Geometry check sheet. Reference: the model listing, model coordinates, mm. Face numbers are marked on the shaded views. A direction names the side the tool comes from. Coordinates: 2 decimals unless noted, no trailing zeros. Write each loop counter-clockwise with the first axis right and the second up, starting at its lowest first coordinate (ties: lowest second). Pieces come first, ordered by that corner, then holes. Notation, with made-up numbers: (49.25, 85) -> (58.25, 85) arc R13 ccw to (58.25, 90) -> close; hole circle Ø11 at (-34, 45.5). An arc over 180 degrees is marked (long way). Answer in a Markdown table with one row per item. Add a question column.
1. Set-up check for the marked faces 1, 2, 3, 4 and 5: record each of +Z, -Z, +X, -X, +Y, -Y from which the full face is reachable in a straight line by a thin tool's end or side.
2. Depth check by flat-ended pin: P1, Ø2, axis at x = 19, z = -17, coming from the -Y side; P2, Ø5.5, axis at x = 6.5, z = -15, coming from the +Y side; P3, Ø1.8, axis at x = -30, z = -1, coming from the +Y side; P4, Ø4, axis at y = -35.36, z = -35.36, coming from the +X side. Enter the tip coordinate at first touch or a pass-through.
3. Cross-section at D-D on y = 22. Record the cut outline in (x, z).
4. Cross-section at B-B on x = 175.7. Record the cut outline in (y, z), and give its area (3 significant figures).
5. Scan lines: L1, parallel to X at y = 43, z = 0; L2, parallel to X at y = 50.5, z = 0; L3, parallel to Z at x = 128.5, y = 24. Record each from-to range of solid material in increasing order. Write a range as from..to.
6. Cross-section at C-C on y = -27. Record the cut outline in (x, z), and give its area (3 significant figures).
7. Cross-section at A-A on z = -19. Record the cut outline in (x, y), and give its area (3 significant figures).
8. Mould release check, pull along X, two halves, no side actions. Record for the marked faces 6, 7 and 8: pulls with the +X half, pulls with the -X half, needs draft (parallel to the pull), parting line crosses it, or undercut.
```python
from build123d import *

# Parameters (mm, degrees)
BOSS_EXTRUDE1_DEPTH      = 10
BOSS_EXTRUDE1_DEPTH_BACK = 38
SKETCH1_3_R              = 40
BOSS_EXTRUDE2_DEPTH      = 10
SKETCH1_4_R              = 45
SKETCH1_4_R_2            = 40
BOSS_EXTRUDE3_DEPTH      = 9
SKETCH2_R                = 45
SKETCH2_W                = 60
SKETCH2_H                = 60
BOSS_EXTRUDE4_DEPTH      = 30
SKETCH2_3_W              = 60
SKETCH2_3_H              = 60
BOSS_EXTRUDE5_DEPTH      = 205.7
SKETCH3_W                = 60
SKETCH3_H                = 60
SKETCH3_R                = 7
BOSS_EXTRUDE6_DEPTH      = 60.5
CHAMFER1_SIZE            = 25
BOSS_EXTRUDE7_DEPTH      = 11
SKETCH7_R                = 3.25
CUT_EXTRUDE2_DEPTH       = 51


with BuildPart() as part:
    # Sketch1 → Boss-Extrude1 (new, two sides: drawn at the far end of the back side and taken through both)
    with BuildSketch(Plane(origin=(0, 0, 0), x_dir=(0, 0, -1), z_dir=(1, 0, 0)).offset(-BOSS_EXTRUDE1_DEPTH_BACK)):
        with BuildLine():
            ThreePointArc((11, 0), (8.774964387, 6.633249581), (3, 10.583005244))
            Line((3, 10.583005244), (3, 8.5))
            Line((3, 8.5), (-3, 8.5))
            Line((-3, 8.5), (-3, 10.583005244))
            ThreePointArc((-3, 10.583005244), (-6.633249581, -8.774964387), (11, 0))
        make_face()
        with BuildLine():
            Line((3, 8.5), (3, 10.583005244))
            ThreePointArc((3, 10.583005244), (0, 11), (-3, 10.583005244))
            Line((-3, 10.583005244), (-3, 8.5))
            Line((-3, 8.5), (3, 8.5))
        make_face()
        with BuildLine():
            Line((3, 10.583005244), (3, 13.5))
            Line((3, 13.5), (-3, 13.5))
            Line((-3, 13.5), (-3, 10.583005244))
            ThreePointArc((-3, 10.583005244), (0, 11), (3, 10.583005244))
        make_face()
    extrude(amount=BOSS_EXTRUDE1_DEPTH + BOSS_EXTRUDE1_DEPTH_BACK)

    # Sketch1_3 → Boss-Extrude2 (add)
    with BuildSketch(Plane(origin=(0, 0, 0), x_dir=(0, 0, -1), z_dir=(1, 0, 0))):
        Circle(SKETCH1_3_R)
        with BuildLine():
            Line((-3, 13.5), (3, 13.5))
            Line((3, 13.5), (3, 10.583005244))
            ThreePointArc((3, 10.583005244), (8.774964387, 6.633249581), (11, 0))
            ThreePointArc((11, 0), (-6.633249581, -8.774964387), (-3, 10.583005244))
            Line((-3, 10.583005244), (-3, 13.5))
        make_face(mode=Mode.SUBTRACT)
    extrude(amount=-BOSS_EXTRUDE2_DEPTH)



with BuildPart() as body_2:
    # Sketch1_4 → Boss-Extrude3 (new body)
    # profile 1 of 3: a face of its own
    with BuildSketch(Plane(origin=(0, 0, 0), x_dir=(0, 0, -1), z_dir=(1, 0, 0))):
        Circle(SKETCH1_4_R)
        Circle(SKETCH1_4_R_2, mode=Mode.SUBTRACT)
    # profile 2 of 3: a face of its own
    with BuildSketch(Plane(origin=(0, 0, 0), x_dir=(0, 0, -1), z_dir=(1, 0, 0))):
        Circle(SKETCH1_4_R_2)
        with BuildLine():
            Line((-3, 13.5), (3, 13.5))
            Line((3, 13.5), (3, 10.583005244))
            ThreePointArc((3, 10.583005244), (8.774964387, 6.633249581), (11, 0))
            ThreePointArc((11, 0), (-6.633249581, -8.774964387), (-3, 10.583005244))
            Line((-3, 10.583005244), (-3, 13.5))
        make_face(mode=Mode.SUBTRACT)
    # profile 3 of 3: a face of its own
    with BuildSketch(Plane(origin=(0, 0, 0), x_dir=(0, 0, -1), z_dir=(1, 0, 0))):
        with BuildLine():
            Line((3, 10.583005244), (3, 13.5))
            Line((3, 13.5), (-3, 13.5))
            Line((-3, 13.5), (-3, 10.583005244))
            ThreePointArc((-3, 10.583005244), (0, 11), (3, 10.583005244))
        make_face()
    extrude(amount=BOSS_EXTRUDE3_DEPTH)


with BuildPart() as part_1:
    add(part.part)

    add(body_2.part)  # Boss-Extrude4 merges body 2
    # Sketch2 → Boss-Extrude4 (add)
    with BuildSketch(Plane(origin=(0, 0, 0), x_dir=(0, 0, -1), z_dir=(1, 0, 0))):
        Circle(SKETCH2_R)
        Rectangle(SKETCH2_W, SKETCH2_H, mode=Mode.SUBTRACT)
    extrude(amount=BOSS_EXTRUDE4_DEPTH)

    # Sketch2_3 → Boss-Extrude5 (add)
    with BuildSketch(Plane(origin=(0, 0, 0), x_dir=(0, 0, -1), z_dir=(1, 0, 0))):
        Rectangle(SKETCH2_3_W, SKETCH2_3_H)
    extrude(amount=BOSS_EXTRUDE5_DEPTH)

    # Sketch3 → Boss-Extrude6 (add)
    with BuildSketch(Plane(origin=(0, 0, 0), x_dir=(1, 0, 0), z_dir=(0, 1, 0))):
        with Locations((175.7, 0)):
            Rectangle(SKETCH3_W, SKETCH3_H)
        with Locations(Location((175.7, 0, 0), (0, 0, 270))):
            Circle(SKETCH3_R, mode=Mode.SUBTRACT)
    extrude(amount=BOSS_EXTRUDE6_DEPTH)

    # Chamfer1
    chamfer1_edges = [part_1.edges().sort_by_distance(p)[0] for p in [
        (205.7, -30, 0),
    ]]
    chamfer(chamfer1_edges, length=CHAMFER1_SIZE)

    # Sketch6 → Boss-Extrude7 (add)
    with BuildSketch(Plane(origin=(0, 0, 0), x_dir=(0, 0, -1), z_dir=(1, 0, 0))):
        with BuildLine():
            Line((45, 35), (35, 45))
            Line((35, 45), (21.794494718, 45))
            ThreePointArc((21.794494718, 45), (35.355339059, 35.355339059), (45, 21.794494718))
            Line((45, 21.794494718), (45, 35))
        make_face()
        with BuildLine():
            ThreePointArc((45, 21.794494718), (35.355339059, 35.355339059), (21.794494718, 45))
            Line((21.794494718, 45), (-21.794494718, 45))
            ThreePointArc((-21.794494718, 45), (-35.355339059, 35.355339059), (-45, 21.794494718))
            Line((-45, 21.794494718), (-45, -21.794494718))
            ThreePointArc((-45, -21.794494718), (-35.355339059, -35.355339059), (-21.794494718, -45))
            Line((-21.794494718, -45), (21.794494718, -45))
            ThreePointArc((21.794494718, -45), (35.355339059, -35.355339059), (45, -21.794494718))
            Line((45, -21.794494718), (45, 21.794494718))
        make_face()
        with BuildLine():
            ThreePointArc((-45, 21.794494718), (-35.355339059, 35.355339059), (-21.794494718, 45))
            Line((-21.794494718, 45), (-35, 45))
            Line((-35, 45), (-45, 35))
            Line((-45, 35), (-45, 21.794494718))
        make_face()
        with BuildLine():
            ThreePointArc((-21.794494718, -45), (-35.355339059, -35.355339059), (-45, -21.794494718))
            Line((-45, -21.794494718), (-45, -35))
            Line((-45, -35), (-35, -45))
            Line((-35, -45), (-21.794494718, -45))
        make_face()
        with BuildLine():
            Line((45, -35), (45, -21.794494718))
            ThreePointArc((45, -21.794494718), (35.355339059, -35.355339059), (21.794494718, -45))
            Line((21.794494718, -45), (35, -45))
            Line((35, -45), (45, -35))
        make_face()
    extrude(amount=BOSS_EXTRUDE7_DEPTH)

    # Sketch7 → Cut-Extrude2 (cut)
    with BuildSketch(Plane(origin=(0, 0, 0), x_dir=(0, 0, -1), z_dir=(1, 0, 0))):
        with Locations((35.355339059, 35.355339059)):
            Circle(SKETCH7_R)
        with Locations((-35.355339059, 35.355339059)):
            Circle(SKETCH7_R)
        with Locations((35.355339059, -35.355339059)):
            Circle(SKETCH7_R)
        with Locations((-35.355339059, -35.355339059)):
            Circle(SKETCH7_R)
    extrude(amount=CUT_EXTRUDE2_DEPTH, mode=Mode.SUBTRACT)


solid = part_1.part
```
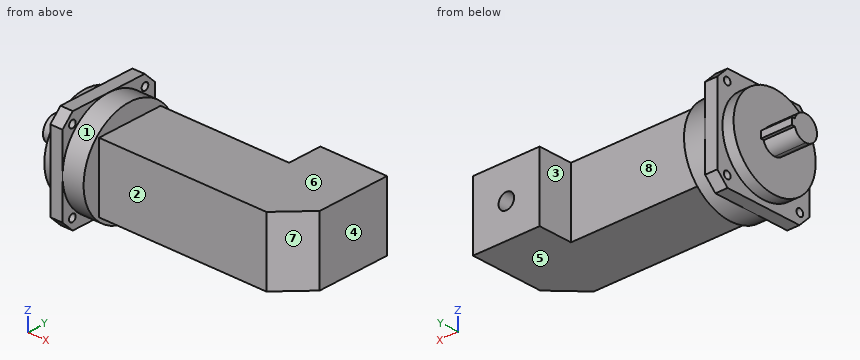
Results found:
| question | item | result |
|---|---|---|
| 1 | face 1 | none |
| 1 | face 2 | +Z, -Z, +X, -Y |
| 1 | face 3 | +Z, -Z, +Y |
| 1 | face 4 | +Z, -Z, +X, +Y, -Y |
| 1 | face 5 | -Z, +X, +Y, -Y |
| 2 | P1 | stops at y = -42.06 |
| 2 | P2 | stops at y = 45 |
| 2 | P3 | stops at y = 13.5 |
| 2 | P4 | passes through |
| 3 | outline | (-10, -33.41) -> (0, -33.41) -> (0, -45) -> (11, -45) -> (11, -39.26) -> (30, -39.26) -> (30, -30) -> (205.7, -30) -> (205.7, 30) -> (30, 30) -> (30, 39.26) -> (11, 39.26) -> (11, 45) -> (0, 45) -> (0, 33.41) -> (-10, 33.41) -> close |
| 4 | outline | (-30, -30) -> (60.5, -30) -> (60.5, -7) -> (30, -7) -> (30, 7) -> (60.5, 7) -> (60.5, 30) -> (-30, 30) -> close |
| 4 | area | 5,000 mm^2 |
| 5 | L1 | x = 0..30, 145.7..168.7, 182.7..205.7 |
| 5 | L2 | x = 145.7..168.7, 182.7..205.7 |
| 5 | L3 | z = -30..30 |
| 6 | outline | (-10, -29.51) -> (0, -29.51) -> (0, -45) -> (11, -45) -> (11, -36) -> (30, -36) -> (30, -30) -> (183.7, -30) -> (183.7, 30) -> (30, 30) -> (30, 36) -> (11, 36) -> (11, 45) -> (0, 45) -> (0, 29.51) -> (-10, 29.51) -> close |
| 6 | area | 12,200 mm^2 |
| 7 | outline | (-10, -35.2) -> (0, -35.2) -> (0, -45) -> (11, -45) -> (11, -40.79) -> (30, -40.79) -> (30, -30) -> (180.7, -30) -> (205.7, -5) -> (205.7, 60.5) -> (145.7, 60.5) -> (145.7, 30) -> (30, 30) -> (30, 40.79) -> (11, 40.79) -> (11, 45) -> (0, 45) -> (0, 35.2) -> (-10, 35.2) -> close |
| 7 | area | 15,300 mm^2 |
| 8 | face 6 | needs draft |
| 8 | face 7 | pulls with the +X half |
| 8 | face 8 | undercut |
